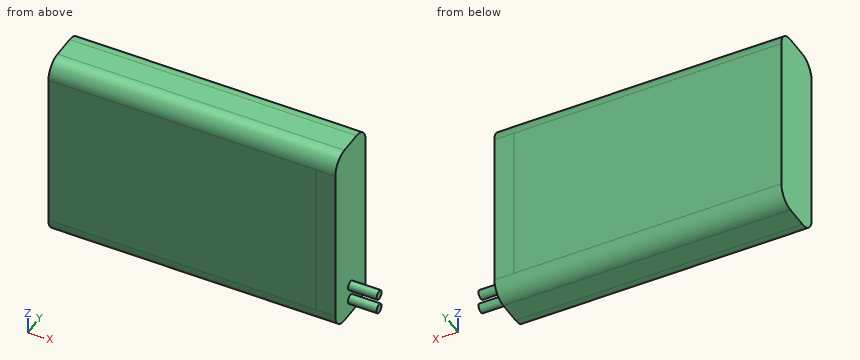
from build123d import *

# Parameters (mm, degrees)
EXTRUDE_2_DEPTH = 50
SKETCH_5_R      = 0.8
EXTRUDE_4_DEPTH = 5
SKETCH_6_R      = 0.8
EXTRUDE_5_DEPTH = 5
SKETCH_7_W      = 3.391372173
SKETCH_7_H      = 28
EXTRUDE_6_DEPTH = 0.0001
SKETCH_8_W      = 3.391372173
SKETCH_8_H      = 28
EXTRUDE_7_DEPTH = 0.0001


with BuildPart() as part:
    # 草图1 → 凸台-拉伸2 (new body)
    with BuildSketch(Plane(origin=(0, 0, 0), x_dir=(0, 0, -1), z_dir=(1, 0, 0))):
        with BuildLine():
            Line((-13.81021057, -5.282067654), (14.18978943, -5.282067654))
            ThreePointArc((14.18978943, -5.282067654), (16.311109773, -4.403387998), (17.18978943, -2.282067654))
            Line((17.18978943, -2.282067654), (17.18978943, 1.717932346))
            ThreePointArc((17.18978943, 1.717932346), (16.311109773, 3.839252689), (14.18978943, 4.717932346))
            Line((14.18978943, 4.717932346), (-13.81021057, 4.717932346))
            ThreePointArc((-13.81021057, 4.717932346), (-15.931530914, 3.839252689), (-16.81021057, 1.717932346))
            Line((-16.81021057, 1.717932346), (-16.81021057, -2.282067654))
            ThreePointArc((-16.81021057, -2.282067654), (-15.931530914, -4.403387998), (-13.81021057, -5.282067654))
        make_face()
    extrude(amount=EXTRUDE_2_DEPTH)

    # 草图5 → 凸台-拉伸4 (add)
    with BuildSketch(Plane(origin=(50, 0, 0), x_dir=(0, 0, -1), z_dir=(1, 0, 0))):
        with Locations(Location((11.628905856, -0.282922759, 0), (0, 0, 180))):
            Circle(SKETCH_5_R)
    extrude(amount=EXTRUDE_4_DEPTH)

    # 草图6 → 凸台-拉伸5 (add)
    with BuildSketch(Plane(origin=(50, 0, 0), x_dir=(0, 0, -1), z_dir=(1, 0, 0))):
        with Locations(Location((14.317760306, -0.301594573, 0), (0, 0, 180))):
            Circle(SKETCH_6_R)
    extrude(amount=EXTRUDE_5_DEPTH)

    # 草图7 → 凸台-拉伸6 (add)
    with BuildSketch(Plane(origin=(0, 4.717932346, 0), x_dir=(1, 0, 0), z_dir=(0, 1, 0))):
        with Locations((48.304313913, 0.18978943)):
            Rectangle(SKETCH_7_W, SKETCH_7_H)
    extrude(amount=EXTRUDE_6_DEPTH)

    # 草图8 → 凸台-拉伸7 (add)
    with BuildSketch(Plane(origin=(0, -5.282067654, 0), x_dir=(-1, 0, 0), z_dir=(0, -1, 0))):
        with Locations((-48.304313913, 0.18978943)):
            Rectangle(SKETCH_8_W, SKETCH_8_H)
    extrude(amount=EXTRUDE_7_DEPTH)


solid = part.part
Geometry: final body of the model. Coordinates: model frame, mm. Give positions to 0.01 mm unless a question says otherwise; leave off trailing zeros. Write each loop counter-clockwise with the first axis right and the second up, starting at its lowest first coordinate (ties: lowest second). Pieces come first, ordered by that corner, then holes. Notation, with made-up numbers: M 55,-28.75 L 107,-28.75 A21 cw 107,5.25 Z; hole C 33.5,57 d1. An arc over 180 degrees is marked long. Answer in a Markdown table with one row per item. Add a question column.
(1) Section B-B on x = 18. Return loops of the section in (y, z), and give its area (3 significant figures).
(2) Section D-D on y = 4. Return loops of the section in (x, z).
(3) Ray query, line 1 (X direction, y = -3, z = -0.5); line 2 (Z direction, x = 10, y = 2); line 3 (Y direction, x = 46, z = 14). Return the intervals inside material, ascending.
(4) Section C-C on y = -3.5. Return loops of the section in (x, z).
Result set:
| question | item | result |
|---|---|---|
| 1 | outline | M -5.28,-14.19 A3 ccw -2.28,-17.19 L 1.72,-17.19 A3 ccw 4.72,-14.19 L 4.72,13.81 A3 ccw 1.72,16.81 L -2.28,16.81 A3 ccw -5.28,13.81 Z |
| 1 | area | 332 mm^2 |
| 2 | outline | M 0,-16.14 L 50,-16.14 L 50,15.76 L 0,15.76 Z |
| 3 | line 1 | x = 0 to 50 |
| 3 | line 2 | z = -17.18 to 16.8 |
| 3 | line 3 | y = -5.28 to 4.71 |
| 4 | outline | M 0,-16.93 L 50,-16.93 L 50,16.55 L 0,16.55 Z |
